The listing builds one solid part. Answer for the finished solid, in the listing's coordinates (mm). A direction names the side the tool comes from. Round coordinates to 2 decimals unless told otherwise and drop trailing zeros. Loops run counter-clockwise (first coordinate to the right, second up) from the corner with the lowest first, then second, coordinate; pieces in that order, holes last. Notation, with made-up numbers: (-35, -22.5) - (-1, -22.5) arc R25 ccw to (-1, -6.5) - close; hole circle Ø5 at (0.25, 41). An arc over 180 degrees is marked (long way). Write item = value, one per line. Start each with the question number.
1) Given pin 1 Ø12 at (x, z) = (16, -18) entering from +Y; pin 2 Ø9 at (x, z) = (0, 0) entering from +Y; pin 3 Ø4 at (y, z) = (10, -1) entering from -X, each flat-ended and moving along its own axis, determine where each tip first touches the part or whether it passes through.
2) Section A-A, the plane z = 0 is taken. Determine the outline of the cut face in (x, y).
3) Section B-B, the plane x = 0 is taken. Determine the outline of the cut face in (y, z).
4) A tool of negligible diameter and unlimited length cuts with its end or side. For faces 5 (the flat face through (0, 15, -8.2)), 6 (the flat face through (17, 0.5, -6)), from which of +Z, -Z, +X, -X, +Y, -Y can it reach the whole face along a straight path? Write none if from no direction.
5) Section C-C, the plane y = 3.25 is taken. Determine the outline of the cut face in (x, z), and give its area (3 significant figures).
6) For a pull along Z with two mould halves and no side action, classify faces 1 (the conical face through (5.215, 12.482, 10.027)), 2 (the cylindrical face through (-1.73, 12.54, 7.81)), 3 (the flat face through (-3.4, 10, 1.7)), 4 (the flat face through (0, -0.5, -6)) as released by +Z, released by -Z, zero draft, split by the parting line, or undercut.
7) Section D-D, the plane x = 20 is taken. Determine the outline of the cut face in (y, z), and give its area (3 significant figures).
8) Straight lines are drawn through the part: line 1 along X through (y, z) = (0, 0); line 2 along Y through (x, z) = (-17.5, 21). For each, find the intervals that lie inside material, in ascending order.
from build123d import *
from build123d.topology import SkipClean

# Parameters (mm, degrees)
BOSS_EXTRUDE1_DEPTH      = 0.5
BOSS_EXTRUDE1_DEPTH_BACK = 0.5
SKETCH1_R                = 3.5


with BuildPart() as part:
    # Sketch1 → Boss-Extrude1 (new, two sides: drawn at the far end of the back side and taken through both)
    with BuildSketch(Plane(origin=(0, 0, 0), x_dir=(1, 0, 0), z_dir=(0, 1, 0)).offset(-BOSS_EXTRUDE1_DEPTH_BACK)):
        with BuildLine():
            Line((-24, 25), (24, 25))
            ThreePointArc((24, 25), (24.707106781, 24.707106781), (25, 24))
            Line((25, 24), (25, -24))
            ThreePointArc((25, -24), (24.707106781, -24.707106781), (24, -25))
            Line((24, -25), (-24, -25))
            ThreePointArc((-24, -25), (-24.707106781, -24.707106781), (-25, -24))
            Line((-25, -24), (-25, 24))
            ThreePointArc((-25, 24), (-24.707106781, 24.707106781), (-24, 25))
        make_face()
        with Locations(Location((0, 0, 0), (0, 0, 270))):
            Circle(SKETCH1_R, mode=Mode.SUBTRACT)
    extrude(amount=BOSS_EXTRUDE1_DEPTH + BOSS_EXTRUDE1_DEPTH_BACK)

    # Sketch2 → Revolve1 (revolve)
    with SkipClean():  # the faces are left unmerged after this step: merging them gives an invalid solid
        with BuildSketch(Plane.XY, mode=Mode.PRIVATE) as revolve1_sk:
            Polygon((-8, 15), (-10, 15), (-17.5, 0.5), (-3.5, 0.5), (-3.5, 10), (-8, 10), align=None)
        revolve(revolve1_sk.sketch.rotate(Axis((0, 0.5, 0), (0, 1, 0)), 180), axis=Axis((0, 0.5, 0), (0, 1, 0)))
    add(part.part.scale(1), mode=Mode.REPLACE)  # the faces are merged on a copy


solid = part.part
Geometry check:
q1.pin_1 = 0.5
q1.pin_2 = 10
q1.pin_3 = -13.59
q2.outline = (-25, -0.5) - (-3.5, -0.5) - (-3.5, 10) - (-8, 10) - (-8, 15) - (-10, 15) - (-17.5, 0.5) - (-25, 0.5) - close; (3.5, -0.5) - (25, -0.5) - (25, 0.5) - (17.5, 0.5) - (10, 15) - (8, 15) - (8, 10) - (3.5, 10) - close
q3.outline = (-0.5, -25) - (0.5, -25) - (0.5, -17.5) - (15, -10) - (15, -8) - (10, -8) - (10, -3.5) - (-0.5, -3.5) - close; (-0.5, 3.5) - (10, 3.5) - (10, 8) - (15, 8) - (15, 10) - (0.5, 17.5) - (0.5, 25) - (-0.5, 25) - close
q4.face_5 = +Z, -Z, +X, -X, +Y
q4.face_6 = +Y
q5.outline = circle Ø32.16 at (0, 0); hole circle Ø7 at (0, 0)
q5.area = 774 mm2
q6.face_1 = split by the parting line
q6.face_2 = undercut
q6.face_3 = undercut
q6.face_4 = zero draft
q7.outline = (-0.5, -25) - (0.5, -25) - (0.5, 25) - (-0.5, 25) - close
q7.area = 50.0 mm2
q8.line_1 = -25 to -3.5, 3.5 to 25
q8.line_2 = -0.5 to 0.5
